Check sheet for the drawn part. Datum: minimum x, y, z corner. Units: mm. A direction names the side the tool comes from. Round coordinates to 2 decimals unless told otherwise and drop trailing zeros. Loops run counter-clockwise (first coordinate to the right, second up) from the corner with the lowest first, then second, coordinate; pieces in that order, holes last.
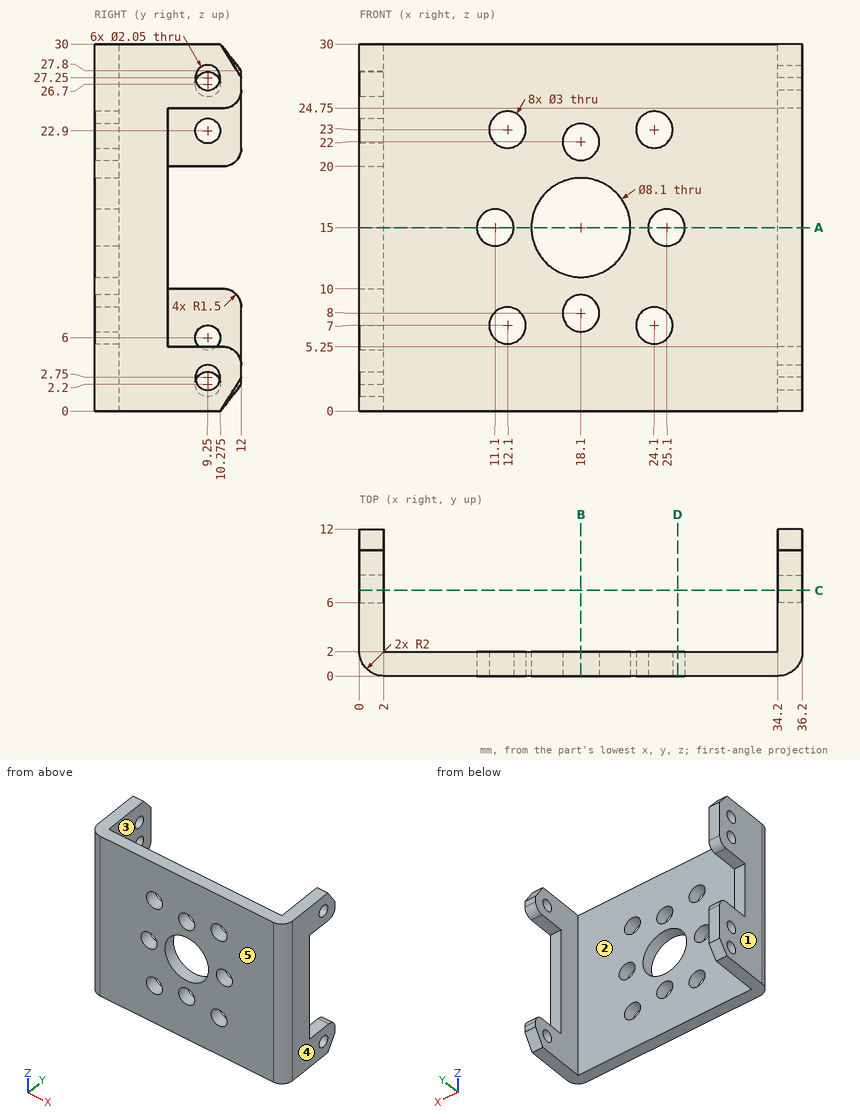
1) Sectioned sample at B-B, the plane x = 18.1. Record the cut outline in (y, z), then the cut area to 3 significant figures.
Report:
outline: (0, 0) - (2, 0) - (2, 6.5) - (0, 6.5) - close; (0, 9.5) - (2, 9.5) - (2, 10.95) - (0, 10.95) - close; (0, 19.05) - (2, 19.05) - (2, 20.5) - (0, 20.5) - close; (0, 23.5) - (2, 23.5) - (2, 30) - (0, 30) - close
area: 31.8 mm2
2) Sectioned sample at D-D, the plane x = 26. Record the cut outline in (y, z), then the cut area to 3 significant figures.
Report:
outline: (0, 0) - (2, 0) - (2, 13.8) - (0, 13.8) - close; (0, 16.2) - (2, 16.2) - (2, 30) - (0, 30) - close
area: 55.2 mm2
3) Access from +Z, -Z, +X, -X, +Y, -Y to the whole of each face (thin tool, end or side, straight path). Record for the marked faces 1 and 2.
Report:
face 1: +Z, -Z, -X, +Y, -Y
face 2: +Z, -Z, +Y
4) Gauge pin test, flat ends, axial feed: pin 1 (2 mm diameter, centred on x = 0.5, z = 15.5, fed in from +Y); pin 2 (5 mm diameter, centred on x = 18.1, z = 8, fed in from +Y); pin 3 (1.2 mm diameter, centred on y = 9.25, z = 2.75, fed in from +X). Record the tip position at first contact, or that the pin passes through.
Report:
pin 1: stops at y = 6
pin 2: stops at y = 2
pin 3: stops at x = 2
5) Mould release check, pull along X, two halves, no side actions. Record for the marked faces 3, 4 and 5: +X half, -X half, draft (parallel to the pull), parting line (faces both ways), or undercut.
Report:
face 3: undercut
face 4: +X half
face 5: draft
6) Sectioned sample at C-C, the plane y = 7. Record the cut outline in (x, z).
Report:
outline: (0, 0) - (2, 0) - (2, 10) - (0, 10) - close; (0, 20) - (2, 20) - (2, 30) - (0, 30) - close; (34.2, 0) - (36.2, 0) - (36.2, 5.25) - (34.2, 5.25) - close; (34.2, 24.75) - (36.2, 24.75) - (36.2, 30) - (34.2, 30) - close
7) Sectioned sample at A-A, the plane z = 15. Record the cut outline in (x, y).
Report:
outline: (0, 2) arc R2 ccw to (2, 0) - (9.6, 0) - (9.6, 2) - (2, 2) - (2, 6) - (0, 6) - close; (12.6, 0) - (14.05, 0) - (14.05, 2) - (12.6, 2) - close; (22.15, 0) - (23.6, 0) - (23.6, 2) - (22.15, 2) - close; (26.6, 0) - (34.2, 0) arc R2 ccw to (36.2, 2) - (36.2, 6) - (34.2, 6) - (34.2, 2) - (26.6, 2) - close
8) Scan lines: line 1 along X through (y, z) = (2.5, 28.75); line 2 along Y through (x, z) = (13, 2). Record each from-to range of solid material in increasing order.
Report:
line 1: x = 0 to 2, 34.2 to 36.2
line 2: y = 0 to 2
